Read the model definition and answer for the solid it produces. Units are mm, in the model's axes. Coordinates: 2 decimals unless noted, no trailing zeros. Order: outer loops, then holes, each group sorted by start corner. A loop starts at its lowest first (then second) coordinate and runs counter-clockwise, first axis right, second up. Notation, with made-up numbers: (50, -31.75) - (64, -31.75) arc R22 cw to (64, -15.75) - close; hole circle Ø1 at (64, -26.75). An arc over 180 degrees is marked (long way). Use one line per item in the form item = value. Start each with the question number.
Autodesk Inventor part; units mm, degrees
ref_plane "YZ Plane" through (0, 0, 0) normal (1, 0, 0) x (0, 1, 0)
ref_plane "XZ Plane" through (0, 0, 0) normal (0, 1, 0) x (-1, 0, 0)
ref_plane "XY Plane" through (0, 0, 0) normal (0, 0, 1) x (1, 0, 0)
sketch "Sketch2" plane through (0, 0, 0) normal (0, 1, 0) x (-1, 0, 0)
  circle A0 centre (0, 0) radius 50
  dimension "d4" = 100
extrude "Extrusion2" add sketch "Sketch2" along normal blind 10
sketch "Sketch3" plane through (0, 10, 0) normal (0, 1, 0) x (1, 0, 0)
  circle A0 centre (0, 0) radius 50
  circle A1 centre (0, 0) radius 47.5
  dimension "d7" = 100
  dimension "d8" = 95
extrude "Extrusion3" add sketch "Sketch3" along normal blind 200
fillet "Fillet1" radius 2 1 edges at (50, 0, 0)
fillet "Fillet2" radius 2 2 edges at (-50, 210, 0) (-47.5, 210, 0)
fillet "Fillet3" radius 2 1 edges at (-47.5, 10, 0)
properties part number "glass" material "Glass"
Q1. For a pull along Z with two mould halves and no side action, classify faces 1 (the cylindrical face through (-10.3, 108.96, -46.37)), 2 (the flat face through (1, 10, 1)), 3 (the flat face through (1, 0, 1)), 4 (the cylindrical face through (3.3, 103.56, 49.89)) as +Z half, -Z half, draft (parallel to the pull), parting line (faces both ways), or undercut.
Q2. Given P1, Ø6, axis at x = -24, z = 37, coming from the +Y side; P2, Ø10, axis at y = 134.5, z = 21.5, coming from the -X side; P3, Ø2, axis at y = 109, z = -21, coming from the -X side, each flat-ended and moving along its own axis, determine where each tip first touches the part or whether it passes through.
Q3. A cutting plane is placed at A-A (y = 125). Give the vertices of the cut face in (x, z), then the cut area to 3 significant figures.
Q4. Consider probe 1 along X at (y, z) = (109, 0); probe 2 along Y at (x, z) = (5.5, 28.5). Determine where each line is inside the solid, lowest interval first.
Result sheet:
q1.face_1 = undercut
q1.face_2 = undercut
q1.face_3 = draft
q1.face_4 = parting line
q2.P1 = 10.8
q2.P2 = -47.2
q2.P3 = -45.83
q3.outline = circle Ø100 at (0, 0); hole circle Ø95 at (0, 0)
q3.area = 766 mm^2
q4.probe_1 = -50 to -47.5, 47.5 to 50
q4.probe_2 = 0 to 10
